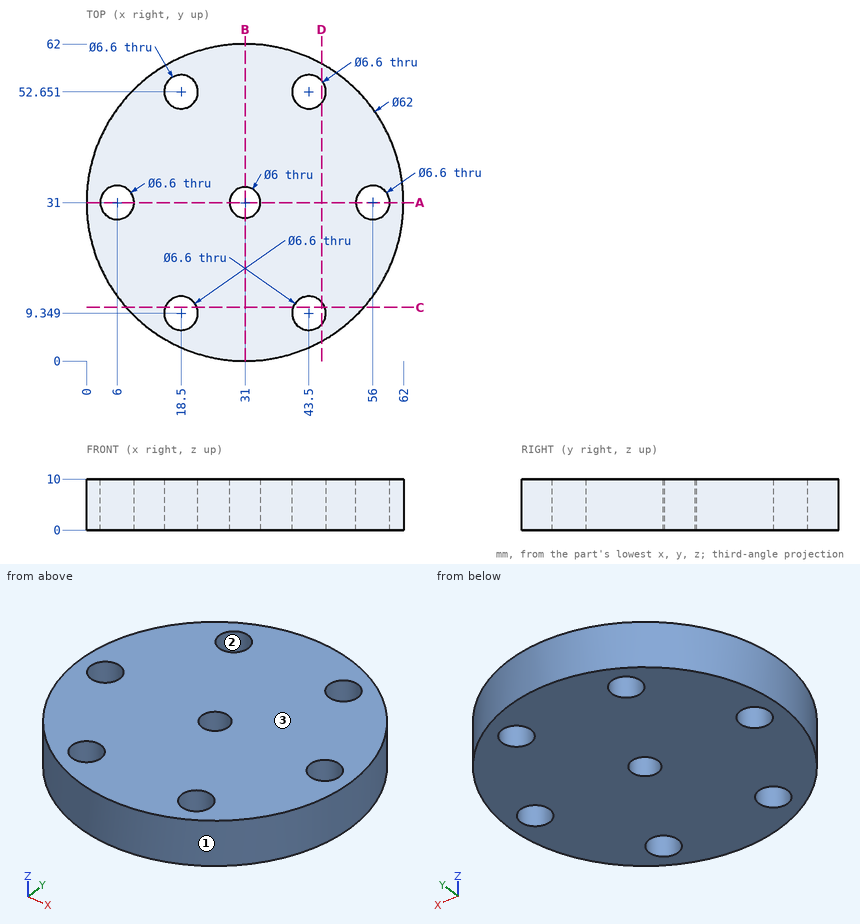
Part print with two shaded views. Sizes in mm from the minimum x, y, z corner. Coordinates: 2 decimals unless noted, no trailing zeros. Write each loop counter-clockwise with the first axis right and the second up, starting at its lowest first coordinate (ties: lowest second). Pieces come first, ordered by that corner, then holes. Notation, with made-up numbers: (36, 39.5) - (84, 39.5) arc R16 cw to (84, 47.5) - close; hole circle Ø2 at (-3, 47.5). An arc over 180 degrees is marked (long way). Use a Markdown table: item, result. Add a question column.
Item 1: Two-plate mould, pull along Y, no slides. Class the marked faces 1, 2 and 3: pulls with the +Y half, pulls with the -Y half, needs draft (parallel to the pull), parting line crosses it, or undercut.
Item 2: Band-saw the part on C-C, the plane y = 10.5. Write the cut outline in (x, z), and give its area (3 significant figures).
Item 3: Drop flat-ended pins along their axis: pin 1 (7.5 mm diameter, centred on x = 6, y = 31, fed in from -Z); pin 2 (5.5 mm diameter, centred on x = 43.5, y = 52.65, fed in from -Z); pin 3 (4 mm diameter, centred on y = 47.5, z = 2, fed in from +X); pin 4 (3 mm diameter, centred on x = 28, z = 3, fed in from +Y). Give the stop position or say it passes through.
Item 4: Band-saw the part on D-D, the plane x = 46. Write the cut outline in (y, z) (1 decimal).
Item 5: Drill centre lines: line 1 along Y through (x, z) = (16.5, 8) (1 decimal); line 2 along Y through (x, z) = (43.5, 5.5); line 3 along Y through (x, z) = (55, 5.75) (1 decimal). Where is each one in solid material? Low to high.
Item 6: Band-saw the part on A-A, the plane y = 31. Write the cut outline in (x, z), and give its area (3 significant figures).
Item 7: Band-saw the part on B-B, the plane x = 31. Write the cut outline in (y, z), and give its area (3 significant figures).
A:
| question | item | result |
|---|---|---|
| 1 | face 1 | parting line crosses it |
| 1 | face 2 | undercut |
| 1 | face 3 | needs draft |
| 2 | outline | (7.75, 0) - (15.41, 0) - (15.41, 10) - (7.75, 10) - close; (21.59, 0) - (40.41, 0) - (40.41, 10) - (21.59, 10) - close; (46.59, 0) - (54.25, 0) - (54.25, 10) - (46.59, 10) - close |
| 2 | area | 341 mm² |
| 3 | pin 1 | stops at z = 0 |
| 3 | pin 2 | passes through |
| 3 | pin 3 | stops at x = 58.4 |
| 3 | pin 4 | stops at y = 61.96 |
| 4 | outline | (3.9, 0) - (7.2, 0) - (7.2, 10) - (3.9, 10) - close; (11.5, 0) - (50.5, 0) - (50.5, 10) - (11.5, 10) - close; (54.8, 0) - (58.1, 0) - (58.1, 10) - (54.8, 10) - close |
| 5 | line 1 | y = 3.6 to 6.7, 12 to 50, 55.3 to 58.4 |
| 5 | line 2 | y = 2.63 to 6.05, 12.65 to 49.35, 55.95 to 59.37 |
| 5 | line 3 | y = 11.4 to 27.9, 34.1 to 50.6 |
| 6 | outline | (0, 0) - (2.7, 0) - (2.7, 10) - (0, 10) - close; (9.3, 0) - (28, 0) - (28, 10) - (9.3, 10) - close; (34, 0) - (52.7, 0) - (52.7, 10) - (34, 10) - close; (59.3, 0) - (62, 0) - (62, 10) - (59.3, 10) - close |
| 6 | area | 428 mm² |
| 7 | outline | (0, 0) - (28, 0) - (28, 10) - (0, 10) - close; (34, 0) - (62, 0) - (62, 10) - (34, 10) - close |
| 7 | area | 560 mm² |
